Geometry: final body of the model. Coordinates: model frame, mm. Face numbers are marked on the shaded views. A direction names the side the tool comes from. Round coordinates to 2 decimals unless told otherwise and drop trailing zeros. Loops run counter-clockwise (first coordinate to the right, second up) from the corner with the lowest first, then second, coordinate; pieces in that order, holes last. Notation, with made-up numbers: M 88,84 L 134,84 A20 ccw 134,100 Z; hole C 14,47.25 d3. An arc over 180 degrees is marked long. Answer as a JSON object with one key per item and string values.
```python
from build123d import *

# Parameters (mm, degrees)
SKETCH_1_R          = 16
EXTRUDE_1_DEPTH     = 7
SKETCH_2_R          = 10
CUT_EXTRUDE_1_DEPTH = 8
SKETCH_3_R          = 14.76
SKETCH_3_R_2        = 11.3
CUT_EXTRUDE_2_DEPTH = 0.5
SKETCH_4_R          = 14.76
SKETCH_4_R_2        = 11.3
CUT_EXTRUDE_3_DEPTH = 0.5


with BuildPart() as part:
    # 草圖1 → 填料-伸長1 (new body)
    with BuildSketch(Plane.XY):
        Circle(SKETCH_1_R)
    extrude(amount=EXTRUDE_1_DEPTH)

    # 草圖2 → 除料-伸長1 (cut, through all)
    with BuildSketch(Plane.XY.offset(7)):
        Circle(SKETCH_2_R)
    extrude(amount=-CUT_EXTRUDE_1_DEPTH, mode=Mode.SUBTRACT)

    # 草圖3 → 除料-伸長2 (cut)
    with BuildSketch(Plane.XY.offset(7)):
        Circle(SKETCH_3_R)
        Circle(SKETCH_3_R_2, mode=Mode.SUBTRACT)
    extrude(amount=-CUT_EXTRUDE_2_DEPTH, mode=Mode.SUBTRACT)

    # 草圖4 → 除料-伸長3 (cut)
    with BuildSketch(Plane(origin=(0, 0, 0), x_dir=(-1, 0, 0), z_dir=(0, 0, -1))):
        Circle(SKETCH_4_R)
        Circle(SKETCH_4_R_2, mode=Mode.SUBTRACT)
    extrude(amount=-CUT_EXTRUDE_3_DEPTH, mode=Mode.SUBTRACT)


solid = part.part
```
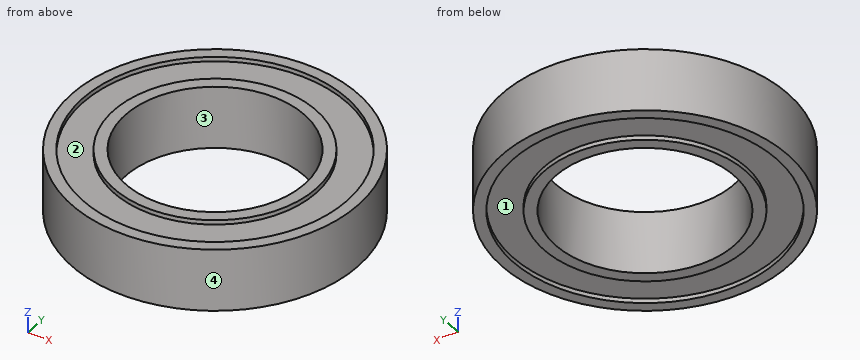
1) Cut plane D-D on z = 2.5. Return the cut outline in (x, y).
Geometry results:
{"outline": "C 0,0 d32; hole C 0,0 d20"}
2) Line query: probe 1 along Y at (x, z) = (0, 6.8); probe 2 along Z at (x, y) = (-9.5, -11); probe 3 along X at (y, z) = (4, 1.25). Output: solid intervals per line, ascending.
Geometry results:
{"probe 1": "-16 to -14.76, -11.3 to -10, 10 to 11.3, 14.76 to 16", "probe 2": "0.5 to 6.5", "probe 3": "-15.49 to -9.17, 9.17 to 15.49"}
3) Set-up query: the marked faces 1 and 2. Return all of +Z, -Z, +X, -X, +Y, -Y with unobstructed straight access to the full face (end or side cutting, diameter ignored); none if empty.
Geometry results:
{"face 1": "-Z", "face 2": "+Z"}
4) Cut plane A-A on y = 0. Return the cut outline in (x, z).
Geometry results:
{"outline": "M -16,0 L -14.76,0 L -14.76,0.5 L -11.3,0.5 L -11.3,0 L -10,0 L -10,7 L -11.3,7 L -11.3,6.5 L -14.76,6.5 L -14.76,7 L -16,7 Z; M 10,0 L 11.3,0 L 11.3,0.5 L 14.76,0.5 L 14.76,0 L 16,0 L 16,7 L 14.76,7 L 14.76,6.5 L 11.3,6.5 L 11.3,7 L 10,7 Z"}
5) Pull-direction query (Y, two-part tool) for the marked faces 3 and 4; classes: +Y half, -Y half, draft (parallel to the pull), parting line (faces both ways), or undercut.
Geometry results:
{"face 3": "undercut", "face 4": "parting line"}
6) Cut plane C-C on x = -12. Return the cut outline in (y, z), and give its area (3 significant figures).
Geometry results:
{"outline": "M -10.58,0 L -8.59,0 L -8.59,0.5 L 8.59,0.5 L 8.59,0 L 10.58,0 L 10.58,7 L 8.59,7 L 8.59,6.5 L -8.59,6.5 L -8.59,7 L -10.58,7 Z", "area": "131 mm2"}
7) First-contact query: pin 1 (2 mm diameter, centred on x = -2.5, z = 3, fed in from +Y); pin 2 (9 mm diameter, centred on x = -1.5, y = -5, fed in from -Z); pin 3 (4 mm diameter, centred on x = 5, z = 0.5, fed in from +Y). Flat tips, straight axial feed; report the tip coordinate or a pass-through.
Geometry results:
{"pin 1": "y = 15.93", "pin 2": "through", "pin 3": "y = 15.72"}
